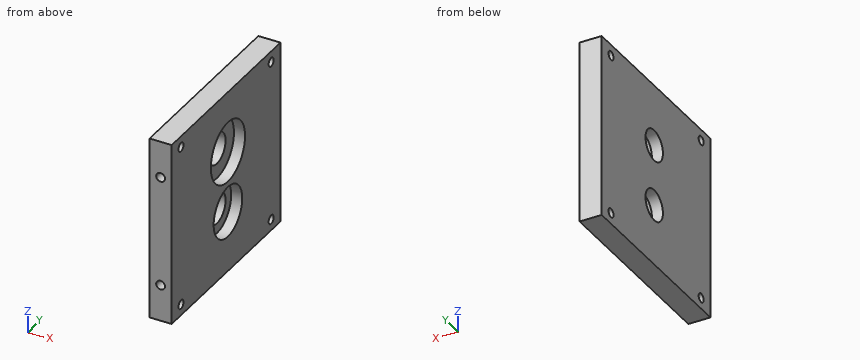
```python
from build123d import *

# Parameters (mm, degrees)
SKETCH1_W           = 20
SKETCH1_H           = 166
BOSS_EXTRUDE1_DEPTH = 175
SKETCH2_R           = 14
CUT_EXTRUDE1_DEPTH  = 175
SKETCH3_R           = 27.5
SKETCH3_R_2         = 23
CUT_EXTRUDE2_DEPTH  = 10
SKETCH4_R           = 4
CUT_EXTRUDE3_DEPTH  = 195.715176604
SKETCH5_R           = 4
CUT_EXTRUDE4_DEPTH  = 15


with BuildPart() as part:
    # Sketch1 → Boss-Extrude1 (new body)
    with BuildSketch(Plane(origin=(0, 0, 0), x_dir=(1, 0, 0), z_dir=(0, 1, 0))):
        Rectangle(SKETCH1_W, SKETCH1_H)
    extrude(amount=BOSS_EXTRUDE1_DEPTH)

    # Sketch2 → Cut-Extrude1 (cut)
    with BuildSketch(Plane(origin=(10, 0, 0), x_dir=(0, 0, -1), z_dir=(1, 0, 0))):
        with Locations((-27.5, 90.5)):
            Circle(SKETCH2_R)
        with Locations((28, 90.5)):
            Circle(SKETCH2_R)
    extrude(amount=-CUT_EXTRUDE1_DEPTH, mode=Mode.SUBTRACT)

    # Sketch3 → Cut-Extrude2 (cut)
    with BuildSketch(Plane(origin=(10, 0, 0), x_dir=(0, 0, -1), z_dir=(1, 0, 0))):
        with Locations((-27.5, 90.5)):
            Circle(SKETCH3_R)
        with Locations((28, 90.5)):
            Circle(SKETCH3_R_2)
    extrude(amount=-CUT_EXTRUDE2_DEPTH, mode=Mode.SUBTRACT)

    # Sketch4 → Cut-Extrude3 (cut, through all)
    with BuildSketch(Plane(origin=(10, 0, 0), x_dir=(0, 0, -1), z_dir=(1, 0, 0))):
        with Locations((73, 160)):
            Circle(SKETCH4_R)
        with Locations(Location((73, 15, 0), (0, 0, 180))):
            Circle(SKETCH4_R)
        with Locations((-73, 15)):
            Circle(SKETCH4_R)
        with Locations(Location((-73, 160, 0), (0, 0, 180))):
            Circle(SKETCH4_R)
    extrude(amount=-CUT_EXTRUDE3_DEPTH, mode=Mode.SUBTRACT)

    # Sketch5 → Cut-Extrude4 (cut)
    with BuildSketch(Plane.XZ):
        with Locations(Location((0, -50, 0), (0, 0, 270))):
            Circle(SKETCH5_R)
        with Locations(Location((0, 50, 0), (0, 0, 90))):
            Circle(SKETCH5_R)
    extrude(amount=-CUT_EXTRUDE4_DEPTH, mode=Mode.SUBTRACT)


solid = part.part
```
Design review of the part built by this model. Coordinates are the model's own, in mm. Give positions to 0.01 mm unless a question says otherwise; leave off trailing zeros. Order: outer loops, then holes, each group sorted by start corner. A loop starts at its lowest first (then second) coordinate and runs counter-clockwise, first axis right, second up. Notation, with made-up numbers: (80.25, -19.5) - (133.25, -19.5) arc R22 ccw to (133.25, 8.5) - close; hole circle Ø10 at (55.25, 71). An arc over 180 degrees is marked (long way). Use a Markdown table: item, result. Add a question column.
(1) Wall thickness on probe 1 along Y at (x, z) = (3, -75.5); probe 2 along X at (y, z) = (4.75, 50); probe 3 along Y at (x, z) = (5, 32.5): over which ranges is each line inside the solid? List them lowest first. Write a range as [from, to].
(2) Add section A-A on z = 27.5. Give the boundary of the cut face in (x, y), then the cut area to 3 significant figures.
(3) Clearance check with flat-ended pins moving along their axes: P1, Ø6.5, axis at x = 0, z = -50, coming from the -Y side; P2, Ø23, axis at y = 81, z = -22, coming from the +X side; P3, Ø17, axis at y = 90.5, z = -28, coming from the -X side. State where each tip first meets the part, or that it passes through.
(4) Add section D-D on x = -6. Give the boundary of the cut face in (y, z), then the cut area to 3 significant figures.
(5) Add section C-C on z = 73. Give the boundary of the cut face in (x, y).
(6) Add section B-B on y = 160. Give the boundary of the cut face in (x, z), then the cut area to 3 significant figures.
Report:
| question | item | result |
|---|---|---|
| 1 | probe 1 | y = [0, 11.88], [18.12, 156.88], [163.12, 175] |
| 1 | probe 2 | x = [-10, -4], [4, 10] |
| 1 | probe 3 | y = [0, 63.46], [117.54, 175] |
| 2 | outline | (-10, 0) - (10, 0) - (10, 63) - (0, 63) - (0, 76.5) - (-10, 76.5) - close; (-10, 104.5) - (0, 104.5) - (0, 118) - (10, 118) - (10, 175) - (-10, 175) - close |
| 2 | area | 2,670 mm² |
| 3 | P1 | stops at y = 15 |
| 3 | P2 | stops at x = 0 |
| 3 | P3 | passes through |
| 4 | outline | (0, -83) - (175, -83) - (175, 83) - (0, 83) - close; hole circle Ø8 at (15, -73); hole circle Ø8 at (15, 73); hole circle Ø28 at (90.5, -28); hole circle Ø28 at (90.5, 27.5); hole circle Ø8 at (160, -73); hole circle Ø8 at (160, 73) |
| 4 | area | 27,600 mm² |
| 5 | outline | (-10, 0) - (10, 0) - (10, 11) - (-10, 11) - close; (-10, 19) - (10, 19) - (10, 156) - (-10, 156) - close; (-10, 164) - (10, 164) - (10, 175) - (-10, 175) - close |
| 6 | outline | (-10, -83) - (10, -83) - (10, -77) - (-10, -77) - close; (-10, -69) - (10, -69) - (10, 69) - (-10, 69) - close; (-10, 77) - (10, 77) - (10, 83) - (-10, 83) - close |
| 6 | area | 3,000 mm² |
